Here's how the part is built. I have some questions about the finished solid (model axes, mm). A direction names the side the tool comes from. Round coordinates to 2 decimals unless told otherwise and drop trailing zeros. Order: outer loops, then holes, each group sorted by start corner. A loop starts at its lowest first (then second) coordinate and runs counter-clockwise, first axis right, second up. Notation, with made-up numbers: (64.25, -3) - (95.25, -3) arc R31 ccw to (95.25, 27) - close; hole circle Ø1 at (36, 73.25). An arc over 180 degrees is marked (long way). One line per item, written item: value.
from build123d import *

# Parameters (mm, degrees)
SKETCH1_R               = 1.1938
BOSS_EXTRUDE1_DEPTH     = 6.4008
SKETCH2_W               = 1.8034
SKETCH2_H               = 7.3406
SKETCH2_W_2             = 1.27
SKETCH2_H_2             = 1.2954
SKETCH2_R               = 0.6985
SKETCH2_W_3             = 1.5494
SKETCH2_H_3             = 0.508
SKETCH2_W_4             = 0.762
CUT_EXTRUDE1_DEPTH      = 20.812
CHAMFER1_SIZE           = 0.1778
BOSS_EXTRUDE3_DEPTH     = 6.4008
SKETCH4_W               = 0.5715
SKETCH4_H               = 7.2038
CUT_EXTRUDE2_DEPTH      = 3.3876
CUT_EXTRUDE2_DEPTH_BACK = 20.812
CUT_EXTRUDE3_DEPTH      = 0.381
CUT_EXTRUDE4_DEPTH      = 0.381
CUT_EXTRUDE5_START      = -0.381
CUT_EXTRUDE5_DEPTH      = 4.4958


with BuildPart() as part:
    # Sketch1 → Boss-Extrude1 (new body)
    with BuildSketch(Plane.XY):
        with BuildLine():
            Line((8.8011, 10.5918), (9.4869, 9.906))
            Line((9.4869, 9.906), (18.796, 9.906))
            ThreePointArc((18.796, 9.906), (19.51442049, 9.60842049), (19.812, 8.89))
            Line((19.812, 8.89), (19.812, 1.016))
            ThreePointArc((19.812, 1.016), (19.51442049, 0.29757951), (18.796, 0))
            Line((18.796, 0), (18.2372, 0))
            Line((18.2372, 0), (18.2372, -7.8486))
            Line((18.2372, -7.8486), (17.653, -7.8486))
            Line((17.653, -7.8486), (17.653, 0))
            Line((17.653, 0), (10.9474, 0))
            Line((10.9474, 0), (10.9474, -7.8486))
            Line((10.9474, -7.8486), (10.3632, -7.8486))
            Line((10.3632, -7.8486), (10.3632, 0))
            Line((10.3632, 0), (2.159, 0))
            Line((2.159, 0), (2.159, -7.8486))
            Line((2.159, -7.8486), (1.5748, -7.8486))
            Line((1.5748, -7.8486), (1.5748, 0))
            Line((1.5748, 0), (1.016, 0))
            ThreePointArc((1.016, 0), (0.29757951, 0.29757951), (0, 1.016))
            Line((0, 1.016), (0, 9.5758))
            ThreePointArc((0, 9.5758), (0.29757951, 10.29422049), (1.016, 10.5918))
            Line((1.016, 10.5918), (6.1595, 10.5918))
            Line((6.1595, 10.5918), (6.1595, 11.574364795))
            ThreePointArc((6.1595, 11.574364795), (6.180021184, 11.643583736), (6.234952941, 11.690433313))
            ThreePointArc((6.234952941, 11.690433313), (7.1628, 11.8872), (8.090647059, 11.690433313))
            ThreePointArc((8.090647059, 11.690433313), (8.145578816, 11.643583736), (8.1661, 11.574364795))
            Line((8.1661, 11.574364795), (8.1661, 10.5918))
            Line((8.1661, 10.5918), (8.8011, 10.5918))
        make_face()
        with Locations((5.1562, 2.8956)):
            Circle(SKETCH1_R, mode=Mode.SUBTRACT)
        with Locations((14.6558, 2.8956)):
            Circle(SKETCH1_R, mode=Mode.SUBTRACT)
    extrude(amount=BOSS_EXTRUDE1_DEPTH)

    # Sketch2 → Cut-Extrude1 (cut, through all)
    with BuildSketch(Plane.ZY):
        with Locations((0.9017, -4.1783)):
            Rectangle(SKETCH2_W, SKETCH2_H)
        with Locations((5.4991, -4.1783)):
            Rectangle(SKETCH2_W, SKETCH2_H)
        with Locations((5.7658, 11.2395)):
            Rectangle(SKETCH2_W_2, SKETCH2_H_2)
        with Locations((3.2004, -6.4516)):
            Circle(SKETCH2_R)
        with Locations((5.6261, -0.254)):
            Rectangle(SKETCH2_W_3, SKETCH2_H_3)
        with Locations((0.7747, -0.254)):
            Rectangle(SKETCH2_W_3, SKETCH2_H_3)
        with Locations((0.381, 11.2395)):
            Rectangle(SKETCH2_W_4, SKETCH2_H_2)
    extrude(amount=-CUT_EXTRUDE1_DEPTH, mode=Mode.SUBTRACT)

    # Chamfer1
    chamfer1_edges = [part.edges().sort_by_distance(p)[0] for p in [
        (1.8669, -7.8486, 1.8034),
        (10.6553, -7.8486, 1.8034),
        (17.9451, -7.8486, 1.8034),
        (18.2372, -7.8486, 3.2004),
        (17.653, -7.8486, 3.2004),
        (10.9474, -7.8486, 3.2004),
        (10.3632, -7.8486, 3.2004),
        (2.159, -7.8486, 3.2004),
        (1.5748, -7.8486, 3.2004),
        (1.8669, -7.8486, 4.5974),
        (10.6553, -7.8486, 4.5974),
        (17.9451, -7.8486, 4.5974),
    ]]
    chamfer(chamfer1_edges, length=CHAMFER1_SIZE)

    # Sketch3 → Boss-Extrude3 (add, through all)
    with BuildSketch(Plane.XY.offset(6.4008)):
        with BuildLine():
            Line((3.2385, 10.5918), (3.2385, 11.7856))
            ThreePointArc((3.2385, 11.7856), (3.387289755, 12.144810245), (3.7465, 12.2936))
            Line((3.7465, 12.2936), (17.7165, 12.2936))
            Line((17.7165, 12.2936), (17.7165, 13.619763092))
            ThreePointArc((17.7165, 13.619763092), (19.6596, 17.7956), (21.6027, 13.619763092))
            Line((21.6027, 13.619763092), (21.6027, 12.2936))
            Line((21.6027, 12.2936), (21.6027, 11.9126))
            Line((21.6027, 11.9126), (3.7465, 11.9126))
            ThreePointArc((3.7465, 11.9126), (3.656697439, 11.875402561), (3.6195, 11.7856))
            Line((3.6195, 11.7856), (3.6195, 10.5918))
            Line((3.6195, 10.5918), (3.2385, 10.5918))
        make_face()
    extrude(amount=-BOSS_EXTRUDE3_DEPTH)

    # Sketch4 → Cut-Extrude2 (cut, two sides)
    with BuildSketch(Plane(origin=(19.812, 0, 0), x_dir=(0, 0, -1), z_dir=(1, 0, 0))) as cut_extrude2_sk:
        with Locations((-0.28575, 14.1937)):
            Rectangle(SKETCH4_W, SKETCH4_H)
        with Locations((-6.11505, 14.1937)):
            Rectangle(SKETCH4_W, SKETCH4_H)
    extrude(amount=CUT_EXTRUDE2_DEPTH, mode=Mode.SUBTRACT)
    extrude(cut_extrude2_sk.sketch, amount=-CUT_EXTRUDE2_DEPTH_BACK, mode=Mode.SUBTRACT)

    # Sketch5 → Cut-Extrude3 (cut)
    with BuildSketch(Plane.XY.offset(5.8293)):
        with BuildLine():
            Line((21.6027, 13.619763092), (21.6027, 15.2556))
            ThreePointArc((21.6027, 15.2556), (19.6596, 17.1987), (17.7165, 15.2556))
            Line((17.7165, 15.2556), (17.7165, 13.619763092))
            ThreePointArc((17.7165, 13.619763092), (19.6596, 17.7956), (21.6027, 13.619763092))
        make_face()
    extrude(amount=-CUT_EXTRUDE3_DEPTH, mode=Mode.SUBTRACT)

    # Sketch6 → Cut-Extrude4 (cut)
    with BuildSketch(Plane(origin=(0, 0, 0.5715), x_dir=(-1, 0, 0), z_dir=(0, 0, -1))):
        with BuildLine():
            Line((-21.6027, 15.2556), (-21.6027, 13.619763092))
            ThreePointArc((-21.6027, 13.619763092), (-19.6596, 17.7956), (-17.7165, 13.619763092))
            Line((-17.7165, 13.619763092), (-17.7165, 15.2556))
            ThreePointArc((-17.7165, 15.2556), (-19.6596, 17.1987), (-21.6027, 15.2556))
        make_face()
    extrude(amount=-CUT_EXTRUDE4_DEPTH, mode=Mode.SUBTRACT)

    # Sketch7 → Cut-Extrude5 (cut)
    with BuildSketch(Plane(origin=(0, 0, 0.5715), x_dir=(-1, 0, 0), z_dir=(0, 0, -1)).offset(CUT_EXTRUDE5_START)):
        with BuildLine():
            Line((-21.6027, 13.619763092), (-21.6027, 12.2936))
            Line((-21.6027, 12.2936), (-17.7165, 12.2936))
            Line((-17.7165, 12.2936), (-17.7165, 13.619763092))
            ThreePointArc((-17.7165, 13.619763092), (-19.6596, 12.7156), (-21.6027, 13.619763092))
        make_face()
    extrude(amount=-CUT_EXTRUDE5_DEPTH, mode=Mode.SUBTRACT)


solid = part.part
Q1. If we section it at C-C, the plane z = 1.25: Please give me the cut outline in (x, y).
Results list:
outline: (0, 1.02) arc R1.02 ccw to (1.02, 0) - (18.8, 0) arc R1.02 ccw to (19.81, 1.02) - (19.81, 8.89) arc R1.02 ccw to (18.8, 9.91) - (9.49, 9.91) - (8.8, 10.59) - (8.17, 10.59) - (8.17, 11.57) arc R0.13 ccw to (8.09, 11.69) arc R2.29 ccw to (6.23, 11.69) arc R0.13 ccw to (6.16, 11.57) - (6.16, 10.59) - (3.62, 10.59) - (3.62, 11.79) arc R0.13 cw to (3.75, 11.91) - (21.6, 11.91) - (21.6, 12.29) - (3.75, 12.29) arc R0.51 ccw to (3.24, 11.79) - (3.24, 10.59) - (1.02, 10.59) arc R1.02 ccw to (0, 9.58) - close; circle Ø5.08 at (19.66, 15.26); hole circle Ø2.39 at (5.16, 2.9); hole circle Ø2.39 at (14.66, 2.9)
Q2. If we section it at A-A, the plane y = -4.25: Please give me the cut outline in (x, z).
Results list:
outline: (1.57, 1.8) - (2.16, 1.8) - (2.16, 4.6) - (1.57, 4.6) - close; (10.36, 1.8) - (10.95, 1.8) - (10.95, 4.6) - (10.36, 4.6) - close; (17.65, 1.8) - (18.24, 1.8) - (18.24, 4.6) - (17.65, 4.6) - close
Q3. If I drill on line 1 along X through (y, z) = (-1.5, 4); line 2 along Y through (x, z) = (14.75, 3.75); line 3 along X through (y, z) = (11, 3.5), over which ranges is the centre line in solid material (lowest first)?
Results list:
line 1: 1.57 to 2.16, 10.36 to 10.95, 17.65 to 18.24
line 2: 0 to 1.71, 4.09 to 9.91, 11.91 to 12.29
line 3: 3.24 to 3.62, 6.16 to 8.17
Q4. If we section it at D-D, the plane x = 12.5: Please give me the cut outline in (y, z).
Results list:
outline: (0, 0) - (9.91, 0) - (9.91, 6.4) - (0, 6.4) - close; (11.91, 0.57) - (12.29, 0.57) - (12.29, 5.83) - (11.91, 5.83) - close
Q5. Will these pins go through, and if not, where does the flat tip stop? pin 1 (2 mm diameter, centred on x = 19, y = 16.5, fed in from +Z); pin 2 (6 mm diameter, centred on x = 15, y = 14, fed in from -Z); pin 3 (1.9 mm diameter, centred on y = 6, z = 4.5, fed in from +X).
Results list:
pin 1: z = 5.83
pin 2: z = 0.57
pin 3: x = 19.81
Q6. If we section it at B-B, the plane x = 8.5: Please give me the cut outline in (y, z), then the cut area to 3 significant figures.
Results list:
outline: (0, 0) - (10.59, 0) - (10.59, 6.4) - (0, 6.4) - close; (11.91, 0.57) - (12.29, 0.57) - (12.29, 5.83) - (11.91, 5.83) - close
area: 69.8 mm²
Q7. Which directions (+Z, -Z, +X, -X, +Y, -Y) give clear straight access to the entire face, cutting with the end or side of a thin tool? Please do faces 5 (the flat face through (7, 11, 5.131)), 6 (the flat face through (13, 12.294, 3)), 7 (the flat face through (20.2, 17.3, 5.448)), 8 (the flat face through (17.653, -4, 3)), 9 (the flat face through (18, 14, 5.829)).
Results list:
face 5: +Z, +X
face 6: -X
face 7: +Z, +Y
face 8: +Z, -Z, -Y
face 9: +Z, +X, -X, +Y
Q8. We'd pull the mould along X, two halves only. Please class faces 1 (the flat face through (10.947, -4, 3)), 2 (the cylindrical face through (19.522, 0.306, 3.156)), 3 (the cylindrical face through (0.306, 0.29, 3.156)), 4 (the flat face through (19.7, 12.5, 0.952)): released by +X, released by -X, zero draft, split by the parting line, or undercut.
Results list:
face 1: undercut
face 2: released by +X
face 3: released by -X
face 4: zero draft
